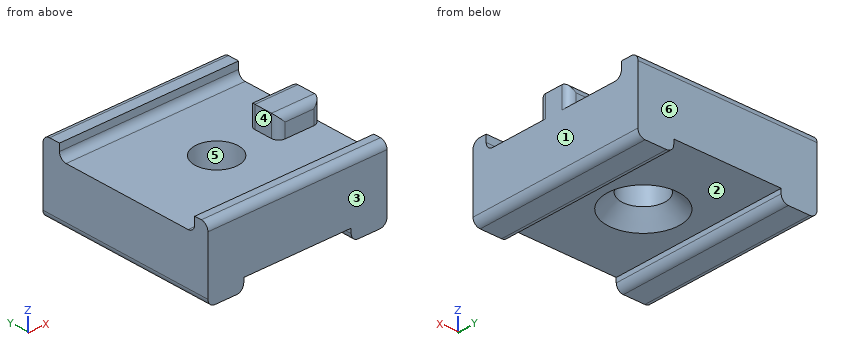
from build123d import *

# Parameters (mm, degrees)
F1_DEPTH = 25
F2_W     = 20.5
F2_H     = 2
F3_DEPTH = 25
F4_R     = 3
F5_DEPTH = 25
F4_W     = 6
F4_H     = 4.5
F6_DEPTH = 3
F7_R     = 1
F8_R     = 1
F9_SIZE  = 2


with BuildPart() as f1:
    # F0 (on Front) → F1 (new body)
    with BuildSketch(Plane.XZ):
        Polygon((14.836072953, 10), (-10.163927047, 10), (-10.163927047, 0), (-5.163927047, 0), (-5.163927047, 1.6477254958), (9.836072953, 1.6477254958), (9.836072953, 0), (14.836072953, 0), align=None)
    extrude(amount=F1_DEPTH)

    # F2 (on face) → F3 (cut)
    with BuildSketch(Plane(origin=(-10.163927047, 0, 0), x_dir=(0, -1, 0), z_dir=(-1, 0, 0))):
        with Locations((12.75, 9)):
            Rectangle(F2_W, F2_H)
    extrude(amount=-F3_DEPTH, mode=Mode.SUBTRACT)

    # F4 (on face) → F5 (cut)
    with BuildSketch(Plane.XY.offset(8)):
        with Locations((2.336072953, -12.75)):
            Circle(F4_R)
    extrude(amount=-F5_DEPTH, mode=Mode.SUBTRACT)

    # F4 (on face) → F6 (join)
    with BuildSketch(Plane.XY.offset(8)):
        with Locations((11.836072953, -12.75)):
            Rectangle(F4_W, F4_H)
    extrude(amount=F6_DEPTH)

    # F7
    f7_edges = [f1.edges().sort_by_distance(p)[0] for p in [
        (11.836073, -10.5, 11),
        (11.836073, -15, 11),
        (8.836073, -10.5, 9.5),
        (8.836073, -15, 9.5),
        (14.836073, -10.5, 9.5),
        (14.836073, -15, 9.5),
    ]]
    fillet(f7_edges, radius=F7_R)

    # F8
    f8_edges = [f1.edges().sort_by_distance(p)[0] for p in [
        (2.336073, -23, 8),
        (2.336073, -2.5, 8),
        (2.336073, -25, 10),
        (2.336073, 0, 10),
        (-10.163927, -12.5, 0),
        (-5.163927, -12.5, 0),
        (9.836073, -12.5, 0),
        (14.836073, -12.5, 0),
    ]]
    fillet(f8_edges, radius=F8_R)

    # F9
    f9_edges = [f1.edges().sort_by_distance(p)[0] for p in [
        (-0.663927, -12.75, 1.647725),
    ]]
    chamfer(f9_edges, length=F9_SIZE)


solid = f1.part
Model file for the job. Use its own axes, mm. Face numbers are marked on the shaded views. A direction names the side the tool comes from. Give positions to 0.01 mm unless a question says otherwise; leave off trailing zeros. Write each loop counter-clockwise with the first axis right and the second up, starting at its lowest first coordinate (ties: lowest second). Pieces come first, ordered by that corner, then holes. Notation, with made-up numbers: M 77,40 L 84,40 A8 cw 84,45 Z; hole C -4,-18 d2. An arc over 180 degrees is marked long. One line per item, written item: value. Start each with the question number.
Q1. Saw through at D-D, the plane z = 2.5. Write the cut outline in (x, y).
Q2. Drop flat-ended pins along their axis: pin 1 Ø12 at (x, y) = (2, -8.5) entering from -Z; pin 2 Ø0.8 at (x, z) = (-3, 9.5) entering from +Y (3 decimals); pin 3 Ø1.2 at (x, y) = (8.5, -2) entering from +Z. Give the stop position or say it passes through.
Q3. Saw through at C-C, the plane y = -19.25. Write the cut outline in (x, z), plus the area to 3 significant figures.
Q4. Probe probe 1 along X at (y, z) = (-4.5, 1.25); probe 2 along X at (y, z) = (-13.5, 7.25); probe 3 along Z at (x, y) = (-5, -20). List the from-to ranges inside material, lowest first. Write a range as [from, to].
Q5. Saw through at B-B, the plane z = 5. Write the cut outline in (x, y).
Q6. 3-axis set-ups, long thin cutter, end or side, ignore diameter. For the marked faces 1 and 2: which of +Z, -Z, +X, -X, +Y, -Y reach the whole face in a straight line?
Q7. Saw through at A-A, the plane y = -12.75. Write the cut outline in (x, z), plus the area to 3 significant figures.
Q8. Two-plate mould, pull along Y, no slides. Class the marked faces 3, 4, 5 and 6: +Y half, -Y half, draft (parallel to the pull), parting line (faces both ways), or undercut.
Output values:
1. outline: M -10.16,-25 L 14.84,-25 L 14.84,0 L -10.16,0 Z; hole C 2.34,-12.75 d8.3
2. pin 1: stops at z = 1.65
2. pin 2: stops at y = -0.005
2. pin 3: stops at z = 10
3. outline: M -10.16,1 A1 ccw -9.16,0 L -6.16,0 A1 ccw -5.16,1 L -5.16,1.65 L 9.84,1.65 L 9.84,1 A1 ccw 10.84,0 L 13.84,0 A1 ccw 14.84,1 L 14.84,8 L -10.16,8 Z
3. area: 174 mm²
4. probe 1: x = [-10.16, -5.16], [9.84, 14.84]
4. probe 2: x = [-10.16, -0.57], [5.24, 14.84]
4. probe 3: z = [1.65, 8]
5. outline: M -10.16,-25 L 14.84,-25 L 14.84,0 L -10.16,0 Z; hole C 2.34,-12.75 d6
6. face 1: +Z, -Z, +X, +Y, -Y
6. face 2: -Z, +Y, -Y
7. outline: M -10.16,1 A1 ccw -9.16,0 L -6.16,0 A1 ccw -5.16,1 L -5.16,1.65 L -2.66,1.65 L -0.66,3.65 L -0.66,8 L -10.16,8 Z; M 5.34,3.65 L 7.34,1.65 L 9.84,1.65 L 9.84,1 A1 ccw 10.84,0 L 13.84,0 A1 ccw 14.84,1 L 14.84,11 L 8.84,11 L 8.84,8 L 5.34,8 Z
7. area: 150 mm²
8. face 3: -Y half
8. face 4: undercut
8. face 5: undercut
8. face 6: +Y half
